Can you work these out from the model? Positions are in its coordinate system, mm. A direction names the side the tool comes from. Give positions to 0.01 mm unless a question says otherwise; leave off trailing zeros. Loops run counter-clockwise (first coordinate to the right, second up) from the corner with the lowest first, then second, coordinate; pieces in that order, holes last. Notation, with made-up numbers: M 28.5,58.25 L 63.5,58.25 A26 cw 63.5,97.25 Z; hole C 1,84.5 d6. An arc over 180 degrees is marked long. Use CSV: the item, a comma, the result in double quotes.
from build123d import *

# Parameters (mm, degrees)
SKETCH008_W         = 75
SKETCH008_H         = 79
PAD003_DEPTH        = 4
SKETCH009_W         = 75
SKETCH009_H         = 15
PAD004_DEPTH        = 6
SKETCH010_R         = 1.6
POCKET005_DEPTH     = 222.779427
SKETCH011_R         = 2.75
POCKET006_DEPTH     = 10.001
SKETCH012_W         = 2.5
SKETCH012_H         = 49
PAD005_DEPTH        = 6
LINEARPATTERN_COUNT = 6
LINEARPATTERN_PITCH = 14.5
SKETCH015_R         = 3.6
POCKET008_DEPTH     = 1.4


with BuildPart() as part:
    # Sketch008 → Pad003 (new body)
    with BuildSketch(Plane.XZ):
        with Locations((-37.5, 39.5)):
            Rectangle(SKETCH008_W, SKETCH008_H)
    extrude(amount=PAD003_DEPTH)

    # Sketch009 (on Face6 of Pad003) → Pad004 (join)
    with BuildSketch(Plane.XZ.offset(4)):
        with Locations((-37.5, 71.5)):
            Rectangle(SKETCH009_W, SKETCH009_H)
        with Locations((-37.5, 7.5)):
            Rectangle(SKETCH009_W, SKETCH009_H)
    extrude(amount=PAD004_DEPTH)

    # Sketch010 (on Face8 of Pad004) → Pocket005 (cut, through all)
    with BuildSketch(Plane.XZ.offset(4)):
        with Locations((-55, 47.5)):
            Circle(SKETCH010_R)
        with Locations((-40, 47.5)):
            Circle(SKETCH010_R)
        with Locations((-40, 31.5)):
            Circle(SKETCH010_R)
        with Locations((-55, 31.5)):
            Circle(SKETCH010_R)
    pocket005 = extrude(amount=-POCKET005_DEPTH, mode=Mode.SUBTRACT)

    # Mirrored: Pocket005 across Sketch010 Axis12
    add(pocket005.mirror(Plane(origin=(-37.5, -4, 64), x_dir=(0, -1, 0), z_dir=(1, 0, 0))), mode=Mode.SUBTRACT)

    # Sketch011 (on Face23 of Mirrored) → Pocket006 (cut, through all)
    with BuildSketch(Plane.XZ.offset(10)):
        with Locations((-67.5, 71.5)):
            Circle(SKETCH011_R)
        with Locations((-7.5, 71.5)):
            Circle(SKETCH011_R)
        with Locations((-7.5, 7.5)):
            Circle(SKETCH011_R)
        with Locations((-67.5, 7.5)):
            Circle(SKETCH011_R)
    extrude(amount=-POCKET006_DEPTH, mode=Mode.SUBTRACT)

    # Sketch012 (on Face8 of Pocket006) → Pad005 (join)
    with BuildSketch(Plane.XZ.offset(4)):
        with Locations((-73.75, 39.5)):
            Rectangle(SKETCH012_W, SKETCH012_H)
    pad005 = extrude(amount=PAD005_DEPTH)

    # LinearPattern: Pad005 ×6
    with Locations(*[(i * LINEARPATTERN_PITCH, 0, 0) for i in range(1, LINEARPATTERN_COUNT)]):
        add(pad005)

    # Sketch015 (on Face25 of LinearPattern) → Pocket008 (cut)
    with BuildSketch(Plane.XZ.offset(10)):
        with Locations((-67.5, 71.5)):
            Circle(SKETCH015_R)
        with Locations((-7.5, 71.5)):
            Circle(SKETCH015_R)
        with Locations((-7.5, 7.5)):
            Circle(SKETCH015_R)
        with Locations((-67.5, 7.5)):
            Circle(SKETCH015_R)
    extrude(amount=-POCKET008_DEPTH, mode=Mode.SUBTRACT)


solid = part.part
Q1. I want a section at B-B, the plane y = -6.5. State how many separate pieces and enclosed holes the cut face has, then the cut area to 3 significant figures.
Model answer:
separate pieces,"1"
enclosed holes,"9"
area,"2,890 mm2"
Q2. I'm going to push flat-ended pins straight in: P1, Ø6, axis at x = -9, z = 71.5, coming from the -Y side; P2, Ø3.5, axis at x = -37.5, z = 49, coming from the -Y side. Where does each tip first touch, or does it pass through?
Model answer:
P1,"y = -10"
P2,"y = -4"
Q3. If we mould it in two halves opening along X, with no side actions, what happens to faces 3 (the flat face through (0, -5, 39)), 4 (the flat face through (-58, -7, 39)), 5 (the flat face through (-38, -5, 79))? For each: released by +X, released by -X, zero draft, split by the parting line, or undercut.
Model answer:
face 3,"released by +X"
face 4,"undercut"
face 5,"zero draft"
Q4. Please list where these lines run through material, in increasing order: L1, parallel to X at y = -4.75, z = 29.5; L2, parallel to Z at x = -55, y = -0.75; L3, parallel to Z at x = -47, y = -6.5. Write a range as from..to.
Model answer:
L1,"-75..-72.5, -60.5..-58, -46..-43.5, -31.5..-29, -17..-14.5, -2.5..0"
L2,"0..29.9, 33.1..45.9, 49.1..79"
L3,"0..15, 64..79"
Q5. I want a section at C-C, the plane x = -35. Please give me the cut outline in (y, z).
Model answer:
outline,"M -10,0 L 0,0 L 0,29.9 L -4,29.9 L -4,15 L -10,15 Z; M -10,64 L -4,64 L -4,49.1 L 0,49.1 L 0,79 L -10,79 Z; M -4,33.1 L 0,33.1 L 0,45.9 L -4,45.9 Z"
Q6. For faces 1 (the flat face through (-46, -7, 39)), 2 (the cylindrical face through (-8.096, -4.36, 4.815)), which set-ups out of +Z, -Z, +X, -X, +Y, -Y let a thin tool reach every point of the face, with its end or its side?
Model answer:
face 1,"-Y"
face 2,"+Y, -Y"
Q7. I want a section at A-A, the plane z = 7.5. Please give me the cut outline in (x, y), then the cut area to 3 significant figures.
Model answer:
outline,"M -75,-10 L -71.1,-10 L -71.1,-8.6 L -70.25,-8.6 L -70.25,0 L -75,0 Z; M -64.75,-8.6 L -63.9,-8.6 L -63.9,-10 L -11.1,-10 L -11.1,-8.6 L -10.25,-8.6 L -10.25,0 L -64.75,0 Z; M -4.75,-8.6 L -3.9,-8.6 L -3.9,-10 L 0,-10 L 0,0 L -4.75,0 Z"
area,"635 mm2"
